```python
from build123d import *

# Parameters (mm, degrees)
ESQUISSE1_W             = 58
ESQUISSE1_H             = 20
EXTRUSION1_DEPTH        = 8
ESQUISSE2_W             = 37.4
ESQUISSE2_H             = 17.4
ENL_V_MAT_EXTRU_1_DEPTH = 6
ESQUISSE3_W             = 9
ESQUISSE3_H             = 4
ENL_V_MAT_EXTRU_2_DEPTH = 21
ESQUISSE4_R             = 2.5
ESQUISSE4_R_2           = 1
ENL_V_MAT_EXTRU_3_DEPTH = 9
ESQUISSE5_R             = 4
EXTRUSION2_DEPTH        = 10
ESQUISSE6_W             = 10.3
ESQUISSE6_H             = 7
ENL_V_MAT_EXTRU_4_DEPTH = 4
ESQUISSE10_W            = 37.4
ESQUISSE10_H            = 0.5
EXTRUSION8_DEPTH        = 20
ESQUISSE8_W             = 3
ESQUISSE8_H             = 15.4
EXTRUSION7_DEPTH        = 6.5
EXTRUSION7_TAPER        = 9
ESQUISSE11_R            = 6
EXTRUSION9_DEPTH        = 2


with BuildPart() as part:
    # Esquisse1 → Extrusion1 (new body)
    with BuildSketch(Plane.XY):
        with Locations((29, 10)):
            Rectangle(ESQUISSE1_W, ESQUISSE1_H)
    extrude(amount=EXTRUSION1_DEPTH)

    # Esquisse2 → Enlèv. mat.-Extru.1 (cut)
    with BuildSketch(Plane(origin=(0, 0, 0), x_dir=(-1, 0, 0), z_dir=(0, 0, -1))):
        with Locations((-29, 10)):
            Rectangle(ESQUISSE2_W, ESQUISSE2_H)
    extrude(amount=-ENL_V_MAT_EXTRU_1_DEPTH, mode=Mode.SUBTRACT)

    # Esquisse3 → Enlèv. mat.-Extru.2 (cut, through all)
    with BuildSketch(Plane(origin=(0, 20, 0), x_dir=(1, 0, 0), z_dir=(0, 1, 0))):
        with Locations((4.5, -6)):
            Rectangle(ESQUISSE3_W, ESQUISSE3_H)
        with Locations((53.5, -6)):
            Rectangle(ESQUISSE3_W, ESQUISSE3_H)
    extrude(amount=-ENL_V_MAT_EXTRU_2_DEPTH, mode=Mode.SUBTRACT)

    # Esquisse4 → Enlèv. mat.-Extru.3 (cut, through all)
    with BuildSketch(Plane(origin=(0, 0, 0), x_dir=(-1, 0, 0), z_dir=(0, 0, -1))):
        with Locations((-53.5, 15)):
            Circle(ESQUISSE4_R)
        with Locations((-46.3, 17.3)):
            Circle(ESQUISSE4_R_2)
        with Locations((-46.3, 2.7)):
            Circle(ESQUISSE4_R_2)
        with Locations((-53.5, 5)):
            Circle(ESQUISSE4_R)
        with Locations((-4.5, 5)):
            Circle(ESQUISSE4_R)
        with Locations((-11.7, 2.7)):
            Circle(ESQUISSE4_R_2)
        with Locations((-11.7, 17.3)):
            Circle(ESQUISSE4_R_2)
        with Locations((-4.5, 15)):
            Circle(ESQUISSE4_R)
    extrude(amount=-ENL_V_MAT_EXTRU_3_DEPTH, mode=Mode.SUBTRACT)

    # Esquisse5 → Extrusion2 (add)
    with BuildSketch(Plane.XY.offset(8)):
        with Locations((19, 10)):
            Circle(ESQUISSE5_R)
    extrude(amount=EXTRUSION2_DEPTH)

    # Esquisse6 → Enlèv. mat.-Extru.4 (cut)
    with BuildSketch(Plane(origin=(0, 0, 0), x_dir=(-1, 0, 0), z_dir=(0, 0, -1))):
        with Locations((-5.15, 10)):
            Rectangle(ESQUISSE6_W, ESQUISSE6_H)
    extrude(amount=-ENL_V_MAT_EXTRU_4_DEPTH, mode=Mode.SUBTRACT)

    # Esquisse10 → Extrusion8 (add)
    with BuildSketch(Plane(origin=(0, 20, 0), x_dir=(1, 0, 0), z_dir=(0, 1, 0))):
        with Locations((29, -6.25)):
            Rectangle(ESQUISSE10_W, ESQUISSE10_H)
    extrude(amount=-EXTRUSION8_DEPTH)

    # Esquisse8 → Extrusion7 (add)
    with BuildSketch(Plane(origin=(0, 0, 0), x_dir=(-1, 0, 0), z_dir=(0, 0, -1))):
        with Locations((-23.806848388, 10)):
            Rectangle(ESQUISSE8_W, ESQUISSE8_H)
        with Locations((-45.489222367, 10)):
            Rectangle(ESQUISSE8_W, ESQUISSE8_H)
        with Locations((-40.088484526, 10)):
            Rectangle(ESQUISSE8_W, ESQUISSE8_H)
        with Locations((-34.193151612, 10)):
            Rectangle(ESQUISSE8_W, ESQUISSE8_H)
        with Locations((-29, 10)):
            Rectangle(ESQUISSE8_W, ESQUISSE8_H)
        with Locations((-17.911515474, 10)):
            Rectangle(ESQUISSE8_W, ESQUISSE8_H)
        with Locations((-12.510777633, 10)):
            Rectangle(ESQUISSE8_W, ESQUISSE8_H)
    extrude(amount=-EXTRUSION7_DEPTH, taper=EXTRUSION7_TAPER)

    # Esquisse11 → Extrusion9 (add)
    with BuildSketch(Plane.XY.offset(8)):
        with Locations((19, 10)):
            Circle(ESQUISSE11_R)
    extrude(amount=EXTRUSION9_DEPTH)


solid = part.part
```
Here's how the part is built. I have some questions about the finished solid (model axes, mm). A direction names the side the tool comes from. Coordinates: 2 decimals unless noted, no trailing zeros. Order: outer loops, then holes, each group sorted by start corner. A loop starts at its lowest first (then second) coordinate and runs counter-clockwise, first axis right, second up.
1) We'd pull the mould along X, two halves only. Please class faces 1 (the face through (51.19, 14.04, 1.97)), 2 (the face through (58, 10, 2)), 3 (the face through (0, 3, 2)), 4 (the face through (53, 10, 4)): +X half, -X half, draft (parallel to the pull), parting line (faces both ways), or undercut.
2) Will these pins go through, and if not, where does the flat tip stop? pin 1 (4 mm diameter, centred on x = 32.5, y = 14.5, fed in from +Z); pin 2 (1 mm diameter, centred on x = 9.5, y = 11, fed in from -Z); pin 3 (5 mm diameter, centred on y = 14, z = 10, fed in from -X).
3) Which directions (+Z, -Z, +X, -X, +Y, -Y) give clear straight access to the entire face, cutting with the end or side of a thin tool? Please do faces 5 (the face through (12, 3, 6.5)), 6 (the face through (1, 6.5, 2)), 7 (the face through (10.3, 9.9, 4.3)).
4) I need wall thicknesses on line 1 (Y direction, x = 53.5, z = 1.6); line 2 (Y direction, x = 11.7, z = 7); line 3 (X direction, y = 1.5, z = 1.5). Which ranges of each line are inside material? Lowest first, please.
5) Imagine slicing it at A-A on z = 2.5. State how many separate pieces and enclosed holes the cut face has, and give its area (3 significant figures).
6) Imagine slicing it at B-B on z = 17.25. List the corners of the cut face in (x, y) for me, and give its area (3 significant figures).
Response values:
1. face 1: undercut
1. face 2: +X half
1. face 3: -X half
1. face 4: draft
2. pin 1: stops at z = 8
2. pin 2: stops at z = 4
2. pin 3: stops at x = 9
3. face 5: +Z
3. face 6: +Z, -Z, -X
3. face 7: -Z
4. line 1: y = 0 to 2.5, 7.5 to 12.5, 17.5 to 20
4. line 2: y = 0 to 1.7, 3.7 to 16.3, 18.3 to 20
4. line 3: x = 0 to 10.3, 47.7 to 58
5. separate pieces: 8
5. enclosed holes: 2
5. area: 590 mm2
6. outline: circle Ø8 at (19, 10)
6. area: 50.3 mm2
